```python
from build123d import *

# Parameters (mm, degrees)
SKETCH2_R           = 19
BOSS_EXTRUDE1_DEPTH = 300
SKETCH3_R           = 5
CUT_EXTRUDE1_DEPTH  = 10
SKETCH4_R           = 80
BOSS_EXTRUDE2_DEPTH = 10


with BuildPart() as part:
    # Sketch1 → Revolve1 (revolve)
    with BuildSketch(Plane.XY, mode=Mode.PRIVATE) as revolve1_sk:
        Polygon((-35.7804045, 0), (34.2195955, 0), (34.2195955, 68), (19.2195955, 68), (19.2195955, 63), (24.2195955, 63), (24.2195955, 13), (-25.7804045, 13), (-25.7804045, 63), (-20.7804045, 63), (-20.7804045, 68), (-35.7804045, 68), align=None)
    revolve(revolve1_sk.sketch.rotate(Axis((-140.082607732, 0, 0), (1, 0, 0)), 90), axis=Axis((-140.082607732, 0, 0), (1, 0, 0)))

    # Sketch2 → Boss-Extrude1 (add)
    with BuildSketch(Plane.ZY.offset(35.7804045)):
        with Locations(Location((0, 0, 0), (0, 0, 180))):
            Circle(SKETCH2_R)
    extrude(amount=BOSS_EXTRUDE1_DEPTH)

    # Sketch3 → Cut-Extrude1 (cut)
    with BuildSketch(Plane.ZY.offset(35.7804045)):
        with Locations((27.961616464, 0)):
            Circle(SKETCH3_R)
    extrude(amount=-CUT_EXTRUDE1_DEPTH, mode=Mode.SUBTRACT)

    # Sketch4 → Boss-Extrude2 (add)
    with BuildSketch(Plane.ZY.offset(335.7804045)):
        Circle(SKETCH4_R)
    extrude(amount=BOSS_EXTRUDE2_DEPTH)


solid = part.part
```
For this review, take the finished solid that the model builds, in its own axes (mm). A direction names the side the tool comes from. Round coordinates to 2 decimals unless told otherwise and drop trailing zeros. Write each loop counter-clockwise with the first axis right and the second up, starting at its lowest first coordinate (ties: lowest second). Pieces come first, ordered by that corner, then holes. Notation, with made-up numbers: (-4.5, 47.25) - (11.5, 47.25) arc R19 cw to (11.5, 82.25) - close; hole circle Ø3 at (7, 6). An arc over 180 degrees is marked (long way). Answer as CSV lines item,"result". Start each with the question number.
(1) For line 1 (X direction, y = 37.5, z = 14.5); line 2 (Y direction, x = 20.55, z = 0); line 3 (Z direction, x = -154, y = 1.5), list the stretches that pass through material, from the lowest coordinate up.
(2) Machinability: for faces 1 (the cylindrical face through (-340.71, -78.1, -17.34)), 2 (the flat face through (-335.78, -17, 17)), 3 (the cylindrical face through (-28.39, -67.42, -8.85)), which of the approach directions +Z, -Z, +X, -X, +Y, -Y give a long, thin tool a straight path to every point of the face, cutting with its end or side? Answer none if there is none.
(3) Add section D-D, the plane z = 0. State the section outline as (x, y) points.
(4) Mouldability with a two-part tool opening along Z and no side actions: class faces 4 (the flat face through (24.22, -15, -1)), 5 (the flat face through (-35.78, 14, 14)), 6 (the cylindrical face through (26.61, -67.42, -8.85)) as +Z half, -Z half, draft (parallel to the pull), parting line (faces both ways), or undercut.
(5) For pin 1 (10 mm diameter, centred on x = -239.5, y = 20, fed in from +Z); pin 2 (10 mm diameter, centred on x = -160.5, z = -9.5, fed in from -Y); pin 3 (4 mm diameter, centred on x = -67.5, z = 9, fed in from -Y), all flat-tipped, find the tip position at first contact; note any pin that passes through.
(6) Add section C-C, the plane y = 27. State the section outline as (x, z) points, plus the area to 3 significant figures.
(7) Add section B-B, the plane z = 52. State the section outline as (x, y) points, plus the area to 3 significant figures.
From the geometry:
1,line 1,"x = -345.78 to -335.78, -35.78 to -25.78, 24.22 to 34.22"
1,line 2,"y = -68 to -63, -13 to 13, 63 to 68"
1,line 3,"z = -18.94 to 18.94"
2,face 1,"+X, -X"
2,face 2,"none"
2,face 3,"+X"
3,outline,"(-345.78, -80) - (-335.78, -80) - (-335.78, -19) - (-35.78, -19) - (-35.78, -68) - (-20.78, -68) - (-20.78, -63) - (-25.78, -63) - (-25.78, -13) - (24.22, -13) - (24.22, -63) - (19.22, -63) - (19.22, -68) - (34.22, -68) - (34.22, 68) - (19.22, 68) - (19.22, 63) - (24.22, 63) - (24.22, 13) - (-25.78, 13) - (-25.78, 63) - (-20.78, 63) - (-20.78, 68) - (-35.78, 68) - (-35.78, 19) - (-335.78, 19) - (-335.78, 80) - (-345.78, 80) - close"
4,face 4,"undercut"
4,face 5,"draft"
4,face 6,"parting line"
5,pin 1,"stops at z = 11.66"
5,pin 2,"stops at y = -18.46"
5,pin 3,"stops at y = -17.66"
6,outline,"(-345.78, -75.31) - (-335.78, -75.31) - (-335.78, 75.31) - (-345.78, 75.31) - close; (-35.78, -62.41) - (-20.78, -62.41) - (-20.78, -56.92) - (-25.78, -56.92) - (-25.78, 56.92) - (-20.78, 56.92) - (-20.78, 62.41) - (-35.78, 62.41) - close; (19.22, -62.41) - (34.22, -62.41) - (34.22, 62.41) - (19.22, 62.41) - (19.22, 56.92) - (24.22, 56.92) - (24.22, -56.92) - (19.22, -56.92) - close"
6,area,"4,110 mm²"
7,outline,"(-345.78, -60.79) - (-335.78, -60.79) - (-335.78, 60.79) - (-345.78, 60.79) - close; (-35.78, -43.82) - (-20.78, -43.82) - (-20.78, -35.57) - (-25.78, -35.57) - (-25.78, 35.57) - (-20.78, 35.57) - (-20.78, 43.82) - (-35.78, 43.82) - close; (19.22, -43.82) - (34.22, -43.82) - (34.22, 43.82) - (19.22, 43.82) - (19.22, 35.57) - (24.22, 35.57) - (24.22, -35.57) - (19.22, -35.57) - close"
7,area,"3,130 mm²"
